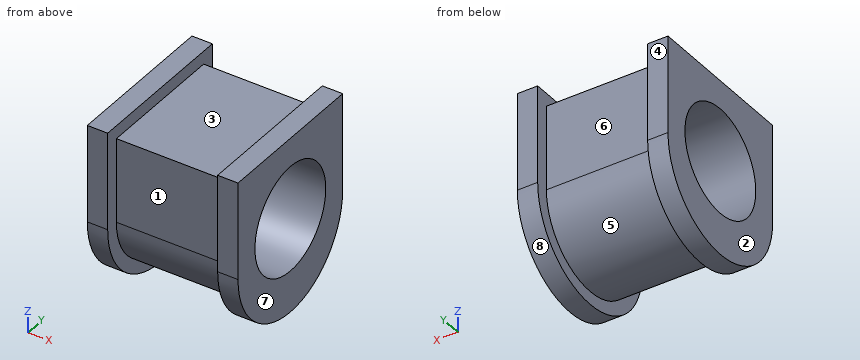
from build123d import *

# Parameters (mm, degrees)
BOSS_EXTRUDE1_DEPTH = 80
BOSS_EXTRUDE2_DEPTH = 12.5
CUT_EXTRUDE1_REACH  = 94.5
SKETCH3_R           = 32.5


with BuildPart() as part:
    # Sketch1 → Boss-Extrude1 (new body)
    with BuildSketch(Plane(origin=(0, 0, 0), x_dir=(0, 0, -1), z_dir=(1, 0, 0))):
        with BuildLine():
            Line((0, 0), (52, 0))
            ThreePointArc((52, 0), (92, 40), (52, 80))
            Line((52, 80), (0, 80))
            Line((0, 80), (0, 0))
        make_face()
    extrude(amount=BOSS_EXTRUDE1_DEPTH)

    # Sketch2 → Boss-Extrude2 (add)
    with BuildSketch(Plane(origin=(80, 0, 0), x_dir=(0, 0, -1), z_dir=(1, 0, 0))):
        with BuildLine():
            Line((-8, 88), (-8, -8))
            Line((-8, -8), (52, -8))
            ThreePointArc((52, -8), (100, 40), (52, 88))
            Line((52, 88), (-8, 88))
        make_face()
    boss_extrude2 = extrude(amount=BOSS_EXTRUDE2_DEPTH)

    # Mirror1: Boss-Extrude2 across plane
    add(boss_extrude2.mirror(Plane(origin=(46.25, 0, 0), x_dir=(0, 0, 1), z_dir=(1, 0, 0))))

    # Sketch3 → Cut-Extrude1 (cut, up to next)
    with BuildSketch(Plane(origin=(92.5, 0, 0), x_dir=(0, 0, -1), z_dir=(1, 0, 0)), mode=Mode.PRIVATE) as cut_extrude1_sk1:
        with Locations((42, 40)):
            Circle(SKETCH3_R)
    cut_extrude1_tool1 = extrude(cut_extrude1_sk1.sketch, amount=-CUT_EXTRUDE1_REACH, mode=Mode.PRIVATE) & part.part
    add(cut_extrude1_tool1.solids().sort_by_distance((92.5, 40, -42))[0], mode=Mode.SUBTRACT)


solid = part.part
For this review, take the finished solid that the model builds, in its own axes (mm). Face numbers are marked on the shaded views. A direction names the side the tool comes from. Give positions to 0.01 mm unless a question says otherwise; leave off trailing zeros. Loops run counter-clockwise (first coordinate to the right, second up) from the corner with the lowest first, then second, coordinate; pieces in that order, holes last.
Item 1: Insertion check: pin 1 (10 mm diameter, centred on x = 38, y = 72.5, fed in from -Z); pin 2 (12 mm diameter, centred on x = 73, y = 55, fed in from -Z); pin 3 (5 mm diameter, centred on x = 73, y = 41.5, fed in from +Z). Each pin has a flat end and moves straight along its axis. Give the tip position at first contact, or say it passes through.
Item 2: Draft analysis for pull direction X (two halves, no side actions). For the marked faces 6, 7 and 8, state which applies: +X half, -X half, draft (parallel to the pull), parting line (faces both ways), or undercut.
Item 3: Take a section at C-C, the plane x = 56. State the section outline as (y, z) points.
Item 4: Take a section at A-A, the plane y = 40. State the section outline as (x, z) points, and give its area (3 significant figures).
Item 5: Tool access review of the marked faces 1, 2, 3, 4 and 5: name each direction out of +Z, -Z, +X, -X, +Y, -Y from which nothing blocks a thin tool from reaching the whole face with its end or side.
Item 6: Take a section at B-B, the plane z = -42. State the section outline as (x, y) points, and give its area (3 significant figures).
Item 7: Take a section at D-D, the plane z = -6. State the section outline as (x, y) points.
Item 8: For line 1 along Y through (x, z) = (44, -42); line 2 along X through (y, z) = (72, 3); line 3 along Z through (x, y) = (76.5, 39), list the stretches that pass through material, from the lowest coordinate up.
Calculated:
1. pin 1: stops at z = -81.05
1. pin 2: stops at z = -90.97
1. pin 3: stops at z = 0
2. face 6: undercut
2. face 7: +X half
2. face 8: draft
3. outline: (0, -52) arc R40 ccw to (80, -52) - (80, 0) - (0, 0) - close; hole circle Ø65 at (40, -42)
4. outline: (0, -100) - (12.5, -100) - (12.5, -92) - (80, -92) - (80, -100) - (92.5, -100) - (92.5, -74.5) - (0, -74.5) - close; (0, -9.5) - (92.5, -9.5) - (92.5, 8) - (80, 8) - (80, 0) - (12.5, 0) - (12.5, 8) - (0, 8) - close
4. area: 2,900 mm2
5. face 1: +Z, -Z, -Y
5. face 2: +Z, -Z, -X, +Y, -Y
5. face 3: +Z, +Y, -Y
5. face 4: +Z, -Z, +X, -X, +Y
5. face 5: -Z
6. outline: (0, -8) - (12.5, -8) - (12.5, 0) - (80, 0) - (80, -8) - (92.5, -8) - (92.5, 7.5) - (0, 7.5) - close; (0, 72.5) - (92.5, 72.5) - (92.5, 88) - (80, 88) - (80, 80) - (12.5, 80) - (12.5, 88) - (0, 88) - close
6. area: 1,790 mm2
7. outline: (0, -8) - (12.5, -8) - (12.5, 0) - (80, 0) - (80, -8) - (92.5, -8) - (92.5, 88) - (80, 88) - (80, 80) - (12.5, 80) - (12.5, 88) - (0, 88) - close
8. line 1: y = 0 to 7.5, 72.5 to 80
8. line 2: x = 0 to 12.5, 80 to 92.5
8. line 3: z = -91.99 to -74.48, -9.52 to 0
